from build123d import *

# Parameters (mm, degrees)
SKETCH1_W               = 47.371
SKETCH1_H               = 29.972
SKETCH1_W_2             = 18.415
SKETCH1_H_2             = 12
BOSS_EXTRUDE1_DEPTH     = 5.08
SKETCH2_W               = 10.11
SKETCH2_H               = 4.63
BOSS_EXTRUDE2_DEPTH     = 2
SKETCH3_W               = 16.045
SKETCH3_H               = 12
CUT_EXTRUDE1_DEPTH      = 6.08
CUT_EXTRUDE1_DEPTH_BACK = 3


with BuildPart() as part:
    # Sketch1 → Boss-Extrude1 (new body)
    with BuildSketch(Plane(origin=(0, 0, 0), x_dir=(1, 0, 0), z_dir=(0, 1, 0))):
        with Locations((23.6855, 0)):
            Rectangle(SKETCH1_W, SKETCH1_H)
        with Locations((-9.2075, 0)):
            Rectangle(SKETCH1_W_2, SKETCH1_H_2)
    extrude(amount=BOSS_EXTRUDE1_DEPTH)

    # Sketch2 → Boss-Extrude2 (add)
    with BuildSketch(Plane(origin=(0, 0, 0), x_dir=(1, 0, 0), z_dir=(0, 1, 0))):
        with Locations((14.855, -12.671)):
            Rectangle(SKETCH2_W, SKETCH2_H)
    extrude(amount=-BOSS_EXTRUDE2_DEPTH)

    # Sketch3 → Cut-Extrude1 (cut, two sides)
    with BuildSketch(Plane(origin=(0, 0, 0), x_dir=(1, 0, 0), z_dir=(0, 1, 0))) as cut_extrude1_sk:
        with Locations((-10.3925, 0)):
            Rectangle(SKETCH3_W, SKETCH3_H)
    extrude(amount=CUT_EXTRUDE1_DEPTH, mode=Mode.SUBTRACT)
    extrude(cut_extrude1_sk.sketch, amount=-CUT_EXTRUDE1_DEPTH_BACK, mode=Mode.SUBTRACT)


solid = part.part
Input: part model. Units: mm. Frame: model coordinates. A direction names the side the tool comes from. Round coordinates to 2 decimals unless told otherwise and drop trailing zeros. Order: outer loops, then holes, each group sorted by start corner. A loop starts at its lowest first (then second) coordinate and runs counter-clockwise, first axis right, second up.
1. Material intervals for line 1 (Y direction, x = 15.5, z = 2.5); line 2 (X direction, y = 0.25, z = 12.75); line 3 (X direction, y = -0.5, z = 12), sorted ascending.
The answers:
line 1: y = 0 to 5.08
line 2: x = 0 to 47.37
line 3: x = 9.8 to 19.91
2. Set-up query: faces 1 (the face through (15, -1, 10.356)), 2 (the face through (0, 3, 11)), 3 (the face through (9.8, -1, 13)), 4 (the face through (-1, 3, -6)), 5 (the face through (19.91, -1, 13)). Return all of +Z, -Z, +X, -X, +Y, -Y with unobstructed straight access to the full face (end or side cutting, diameter ignored); none if empty.
The answers:
face 1: -Z, +X, -X, -Y
face 2: +Z, -X, +Y, -Y
face 3: +Z, -Z, -X, -Y
face 4: -Z, -X, +Y, -Y
face 5: +Z, -Z, +X, -Y
3. Cut plane A-A, the plane x = 15.5. Output: boundary loops of the cut face in (y, z).
The answers:
outline: (-2, 10.36) - (0, 10.36) - (0, -14.99) - (5.08, -14.99) - (5.08, 14.99) - (-2, 14.99) - close
4. Cut plane D-D, the plane z = -11. Output: boundary loops of the cut face in (x, y), then the cut area to 3 significant figures.
The answers:
outline: (0, 0) - (47.37, 0) - (47.37, 5.08) - (0, 5.08) - close
area: 241 mm2
5. Cut plane B-B, the plane y = 1.5. Output: boundary loops of the cut face in (x, z).
The answers:
outline: (-2.37, -6) - (0, -6) - (0, -14.99) - (47.37, -14.99) - (47.37, 14.99) - (0, 14.99) - (0, 6) - (-2.37, 6) - close
6. Pin query (flat end, axial travel): P1, Ø0.7, axis at x = -1, y = 2, coming from the -Z side; P2, Ø0.6, axis at y = -1, z = 12.5, coming from the +X side; P3, Ø0.7, axis at x = -1, y = 2, coming from the +Z side. Return the tip coordinate at first contact, or that it passes through.
The answers:
P1: stops at z = -6
P2: stops at x = 19.91
P3: stops at z = 6
7. Cut plane C-C, the plane z = 13.25. Output: boundary loops of the cut face in (x, y).
The answers:
outline: (0, 0) - (9.8, 0) - (9.8, -2) - (19.91, -2) - (19.91, 0) - (47.37, 0) - (47.37, 5.08) - (0, 5.08) - close
